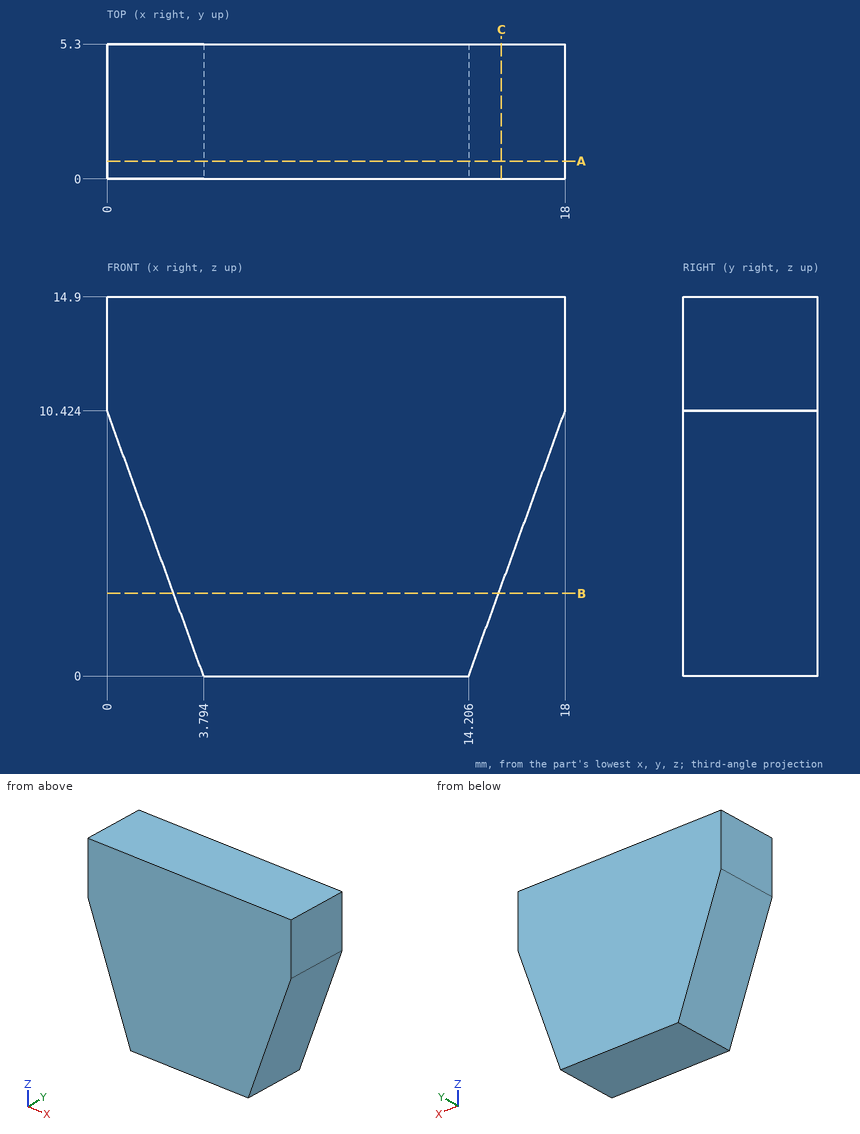
Here's the drawing with two shaded views (mm, measured from the low corner). I have some questions. Round coordinates to 2 decimals unless told otherwise and drop trailing zeros. Write each loop counter-clockwise with the first axis right and the second up, starting at its lowest first coordinate (ties: lowest second). Pieces come first, ordered by that corner, then holes. Notation, with made-up numbers: M -27,69 L 9,69 A31 cw 9,99 Z; hole C 19.5,-4 d6. An arc over 180 degrees is marked long. Write each question's results on one line, items separated by ' | '. Start each with the question number.
1. Imagine slicing it at C-C on x = 15.5. List the corners of the cut face in (y, z) for me.
2. Imagine slicing it at B-B on z = 3.25. List the corners of the cut face in (x, y) for me, and give its area (3 significant figures).
3. Imagine slicing it at A-A on y = 0.7. List the corners of the cut face in (x, z) for me, and give its area (3 significant figures).
4. I need wall thicknesses on L1, parallel to X at y = 2.7, z = 7.25 (1 decimal); L2, parallel to X at y = 3.5, z = 6.5. Which ranges of each line are inside material? Lowest first, please. Write a range as from..to.
Result sheet:
1) outline: M 0,3.56 L 5.3,3.56 L 5.3,14.9 L 0,14.9 Z
2) outline: M 2.61,0 L 15.39,0 L 15.39,5.3 L 2.61,5.3 Z | area: 67.7 mm^2
3) outline: M 0,10.42 L 3.79,0 L 14.21,0 L 18,10.42 L 18,14.9 L 0,14.9 Z | area: 229 mm^2
4) L1: x = 1.2..16.8 | L2: x = 1.43..16.57
